Here's the drawing with two shaded views (mm, measured from the low corner). I have some questions. Coordinates: 2 decimals unless noted, no trailing zeros. Loops run counter-clockwise (first coordinate to the right, second up) from the corner with the lowest first, then second, coordinate; pieces in that order, holes last. Notation, with made-up numbers: (34.25, 1) -> (63.25, 1) arc R31 ccw to (63.25, 29) -> close; hole circle Ø4 at (-6, 51.25). An arc over 180 degrees is marked (long way). Answer as a JSON object with one key per item and string values. Group by question number.
Q1. I want a section at A-A on x = 115. Write out the boundary of the cut face in (y, z).
Q2. I want a section at B-B on z = 5. Write out the boundary of the cut face in (x, y).
Q3. I'm going to push flat-ended pins straight in: pin 1 (2.5 mm diameter, centred on x = 115, z = 5, fed in from -Y); pin 2 (5 mm diameter, centred on x = 115, z = 85, fed in from +Y). Where does each tip first touch, or does it pass through?
Q4. I need wall thicknesses on line 1 (Z direction, x = 115, y = 0.65); line 2 (X direction, y = 0.7, z = 5). Which ranges of each line are inside material? Lowest first, please.
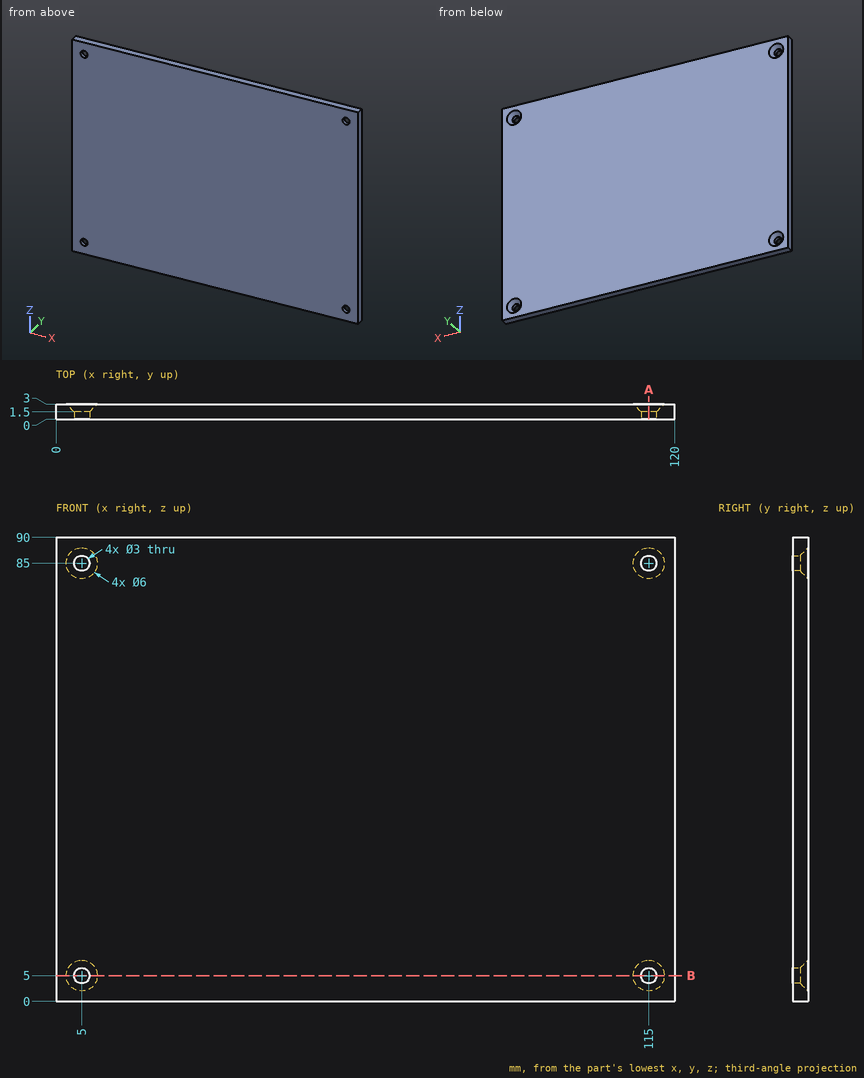
Result set:
{
 "1": {"outline": "(0, 0) -> (3, 0) -> (3, 2) -> (1.5, 3.5) -> (0, 3.5) -> close; (0, 6.5) -> (1.5, 6.5) -> (3, 8) -> (3, 82) -> (1.5, 83.5) -> (0, 83.5) -> close; (0, 86.5) -> (1.5, 86.5) -> (3, 88) -> (3, 90) -> (0, 90) -> close"},
 "2": {"outline": "(0, 0) -> (3.5, 0) -> (3.5, 1.5) -> (2, 3) -> (0, 3) -> close; (6.5, 0) -> (113.5, 0) -> (113.5, 1.5) -> (112, 3) -> (8, 3) -> (6.5, 1.5) -> close; (116.5, 0) -> (120, 0) -> (120, 3) -> (118, 3) -> (116.5, 1.5) -> close"},
 "3": {"pin 1": "passes through", "pin 2": "stops at y = 2.5"},
 "4": {"line 1": "z = 0 to 3.5, 6.5 to 83.5, 86.5 to 90", "line 2": "x = 0 to 3.5, 6.5 to 113.5, 116.5 to 120"}
}
